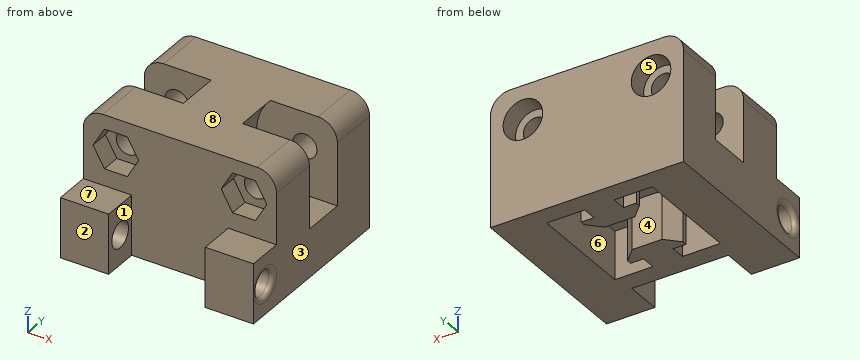
```python
from build123d import *

# Parameters (mm, degrees)
SKETCH1_W           = 40
SKETCH1_H           = 27
BOSS_EXTRUDE1_DEPTH = 30
CUT_EXTRUDE1_DEPTH  = 10
SKETCH3_R           = 2.5
CUT_EXTRUDE2_DEPTH  = 30
CUT_EXTRUDE5_START  = -10.62
CUT_EXTRUDE5_DEPTH  = 9
SKETCH10_W          = 20
SKETCH10_H          = 9
CUT_EXTRUDE7_DEPTH  = 6.8
SKETCH12_W          = 20
SKETCH12_H          = 9
CUT_EXTRUDE10_DEPTH = 6.8
FILLET1_R           = 4
SKETCH13_W          = 12.4
SKETCH13_H          = 7.4
SKETCH13_R          = 2.675
BOSS_EXTRUDE2_DEPTH = 40
CUT_EXTRUDE11_REACH = 42.436
SKETCH14_W          = 20
SKETCH14_H          = 7.4
SKETCH15_R          = 4.1
CUT_EXTRUDE12_DEPTH = 4
SKETCH16_R          = 2.5
CUT_EXTRUDE13_DEPTH = 4
FILLET2_SIZE        = 1


with BuildPart() as part:
    # Sketch1 → Boss-Extrude1 (new body)
    with BuildSketch(Plane(origin=(0, 0, 0), x_dir=(1, 0, 0), z_dir=(0, 1, 0))):
        with Locations((-2.846153846, 4.313186813)):
            Rectangle(SKETCH1_W, SKETCH1_H)
    extrude(amount=BOSS_EXTRUDE1_DEPTH)

    # Sketch2 → Cut-Extrude1 (cut)
    with BuildSketch(Plane(origin=(0, 0, -17.813186813), x_dir=(-1, 0, 0), z_dir=(0, 0, -1))):
        Polygon((-8.086431081, 26), (-8.086431081, 4), (-0.206431081, 4), (-0.206431081, 7), (-2.866431081, 7), (-2.866431081, 8.008707537), (-0.253846154, 10.628707537), (5.946153846, 10.628707537), (8.558738773, 8.008707537), (8.558738773, 7), (5.898738773, 7), (5.898738773, 4), (13.778738773, 4), (13.778738773, 26), (5.898738773, 26), (5.898738773, 23), (8.558738773, 23), (8.558738773, 21.991292463), (5.938738773, 19.378707537), (-0.246431081, 19.378707537), (-2.866431081, 21.991292463), (-2.866431081, 23), (-0.206431081, 23), (-0.206431081, 26), align=None)
    extrude(amount=-CUT_EXTRUDE1_DEPTH, mode=Mode.SUBTRACT)

    # Sketch3 → Cut-Extrude2 (cut)
    with BuildSketch(Plane.XZ):
        with Locations(Location((10.423846154, 2.186813187, 0), (0, 0, 270))):
            Circle(SKETCH3_R)
        with Locations(Location((-16.116153846, 2.186813187, 0), (0, 0, 90))):
            Circle(SKETCH3_R)
    extrude(amount=-CUT_EXTRUDE2_DEPTH, mode=Mode.SUBTRACT)

    # Sketch8 → Cut-Extrude5 (cut)
    with BuildSketch(Plane.XZ.offset(CUT_EXTRUDE5_START)):
        with BuildLine():
            Line((3.282417725, 9.186813187), (17.153846154, 9.186813187))
            Line((17.153846154, 9.186813187), (17.153846154, -7.813186813))
            Line((17.153846154, -7.813186813), (10.423846154, -7.813186813))
            ThreePointArc((10.423846154, -7.813186813), (1.204301697, -1.686170159), (3.282417725, 9.186813187))
        make_face()
        with BuildLine():
            Line((-22.846153846, -7.813186813), (-16.116153846, -7.813186813))
            ThreePointArc((-16.116153846, -7.813186813), (-6.896609389, -1.686170159), (-8.974725418, 9.186813187))
            Line((-8.974725418, 9.186813187), (-22.846153846, 9.186813187))
            Line((-22.846153846, 9.186813187), (-22.846153846, -7.813186813))
        make_face()
    extrude(amount=-CUT_EXTRUDE5_DEPTH, mode=Mode.SUBTRACT)

    # Sketch10 → Cut-Extrude7 (cut)
    with BuildSketch(Plane.ZY.offset(-8.086431081)):
        with Locations((-7.813186813, 15.12)):
            Rectangle(SKETCH10_W, SKETCH10_H)
    extrude(amount=CUT_EXTRUDE7_DEPTH, mode=Mode.SUBTRACT)

    # Sketch12 → Cut-Extrude10 (cut)
    with BuildSketch(Plane(origin=(-13.778738773, 0, 0), x_dir=(0, 0, -1), z_dir=(1, 0, 0))):
        with Locations((7.813186813, 15.12)):
            Rectangle(SKETCH12_W, SKETCH12_H)
    extrude(amount=CUT_EXTRUDE10_DEPTH, mode=Mode.SUBTRACT)

    # Fillet1
    fillet1_edges = [part.edges().sort_by_distance(p)[0] for p in [
        (17.153846154, 24.81, 9.186813187),
        (-22.846153846, 24.81, 9.186813187),
        (17.153846154, 5.31, 9.186813187),
        (-22.846153846, 5.31, 9.186813187),
    ]]
    fillet(fillet1_edges, radius=FILLET1_R)

    # Sketch13 → Boss-Extrude2 (add)
    with BuildSketch(Plane(origin=(17.153846154, 0, 0), x_dir=(0, 0, -1), z_dir=(1, 0, 0))):
        with Locations((11.613186813, -3.7)):
            Rectangle(SKETCH13_W, SKETCH13_H)
        with Locations((11.613186813, -3.7)):
            Circle(SKETCH13_R, mode=Mode.SUBTRACT)
    extrude(amount=-BOSS_EXTRUDE2_DEPTH)

    # Sketch14 → Cut-Extrude11 (cut, up to next)
    with BuildSketch(Plane.XY.offset(-5.413186813), mode=Mode.PRIVATE) as cut_extrude11_sk1:
        with Locations((-2.846153846, -3.7)):
            Rectangle(SKETCH14_W, SKETCH14_H)
    cut_extrude11_tool1 = extrude(cut_extrude11_sk1.sketch, amount=-CUT_EXTRUDE11_REACH, mode=Mode.PRIVATE) & part.part
    add(cut_extrude11_tool1.solids().sort_by_distance((-2.846154, -3.7, -5.413187))[0], mode=Mode.SUBTRACT)

    # Sketch15 → Cut-Extrude12 (cut)
    with BuildSketch(Plane(origin=(0, 30, 0), x_dir=(1, 0, 0), z_dir=(0, 1, 0))):
        with Locations(Location((-16.116153846, -2.186813187, 0), (0, 0, 270))):
            Circle(SKETCH15_R)
        with Locations(Location((10.423846154, -2.186813187, 0), (0, 0, 90))):
            Circle(SKETCH15_R)
    extrude(amount=-CUT_EXTRUDE12_DEPTH, mode=Mode.SUBTRACT)

    # Sketch16 → Cut-Extrude13 (cut)
    # profile 1 of 2: a face of its own
    with BuildSketch(Plane.XZ):
        Polygon((-13.749017742, -1.913186813), (-11.381881639, 2.186813187), (-13.749017742, 6.286813187), (-18.48328995, 6.286813187), (-20.850426054, 2.186813187), (-18.48328995, -1.913186813), align=None)
        with Locations(Location((-16.116153846, 2.186813187, 0), (0, 0, 270))):
            Circle(SKETCH16_R, mode=Mode.SUBTRACT)
    # profile 2 of 2: a face of its own
    with BuildSketch(Plane.XZ):
        Polygon((12.790982258, -1.913186813), (15.158118361, 2.186813187), (12.790982258, 6.286813187), (8.05671005, 6.286813187), (5.689573946, 2.186813187), (8.05671005, -1.913186813), align=None)
        with Locations(Location((10.423846154, 2.186813187, 0), (0, 0, 270))):
            Circle(SKETCH16_R, mode=Mode.SUBTRACT)
    extrude(amount=-CUT_EXTRUDE13_DEPTH, mode=Mode.SUBTRACT)

    # Fillet2
    # a fillet whose section is not a circle: 1 mm, written as the material it takes off along each edge
    with BuildSketch(Plane(origin=(-22.846153846, -3.7, -11.613186813), x_dir=(0, 0, -1), z_dir=(0, -1, 0))) as fillet2_piece_1:
        with BuildLine():
            Bezier((2.675, FILLET2_SIZE), (2.675, 0), (2.675 + FILLET2_SIZE, 0), weights=[1, 1, 1])
            Line((2.675 + FILLET2_SIZE, 0), (2.675, 0))
            Line((2.675, 0), (2.675, FILLET2_SIZE))
        make_face()
    revolve(axis=Axis((-22.846153846, -3.7, -11.613186813), (1, 0, 0)), mode=Mode.SUBTRACT)
    with BuildSketch(Plane(origin=(17.153846154, -3.7, -11.613186813), x_dir=(0, 0, -1), z_dir=(0, -1, 0))) as fillet2_piece_2:
        with BuildLine():
            Bezier((2.675, -FILLET2_SIZE), (2.675, 0), (2.675 + FILLET2_SIZE, 0), weights=[1, 1, 1])
            Line((2.675 + FILLET2_SIZE, 0), (2.675, 0))
            Line((2.675, 0), (2.675, -FILLET2_SIZE))
        make_face()
    revolve(axis=Axis((17.153846154, -3.7, -11.613186813), (1, 0, 0)), mode=Mode.SUBTRACT)


solid = part.part
```
Verification items for the finished model (mm, model axes). Face numbers are marked on the shaded views. A direction names the side the tool comes from. Coordinates: 2 decimals unless noted, no trailing zeros. Loops run counter-clockwise (first coordinate to the right, second up) from the corner with the lowest first, then second, coordinate; pieces in that order, holes last. Notation, with made-up numbers: (5, -35.75) -> (46, -35.75) arc R9 ccw to (46, -31.75) -> close; hole circle Ø11 at (-3.5, -14.75). An arc over 180 degrees is marked (long way). Answer in a Markdown table with one row per item.
1) Section check C-C (y = 5). Record the cut outline in (x, z), and give its area (3 significant figures).
The answers:
| item | result |
|---|---|
| outline | (-22.85, -17.81) -> (-13.78, -17.81) -> (-13.78, -7.81) -> (-5.9, -7.81) -> (-5.9, -17.81) -> (0.21, -17.81) -> (0.21, -7.81) -> (8.09, -7.81) -> (8.09, -17.81) -> (17.15, -17.81) -> (17.15, 5.19) arc R4 ccw to (13.15, 9.19) -> (-18.85, 9.19) arc R4 ccw to (-22.85, 5.19) -> close; hole circle Ø5 at (-16.12, 2.19); hole circle Ø5 at (10.42, 2.19) |
| area | 876 mm2 |
2) Draft check along X on the marked faces 1, 2, 3 and 4. Enter one of: released by +X, released by -X, zero draft, split by the parting line, or undercut.
The answers:
| item | result |
|---|---|
| face 1 | undercut |
| face 2 | zero draft |
| face 3 | released by +X |
| face 4 | undercut |
3) Section check A-A (y = 17). Record the cut outline in (x, z), and give its area (3 significant figures).
The answers:
| item | result |
|---|---|
| outline | (-22.85, -17.81) -> (-13.78, -17.81) -> (-13.78, -7.54) arc R10 cw to (-16.12, -7.81) -> (-22.85, -7.81) -> close; (-8.97, 9.19) arc R10 cw to (-6.98, -1.88) -> (-6.98, -7.81) -> (1.29, -7.81) -> (1.29, -1.88) arc R10 cw to (3.28, 9.19) -> close; (8.09, -17.81) -> (17.15, -17.81) -> (17.15, -7.81) -> (10.42, -7.81) arc R10 cw to (8.09, -7.54) -> close |
| area | 318 mm2 |
4) Section check D-D (z = -2.5). Record the cut outline in (x, y).
The answers:
| item | result |
|---|---|
| outline | (-22.85, 0) -> (17.15, 0) -> (17.15, 10.62) -> (1.29, 10.62) -> (1.29, 19.62) -> (17.15, 19.62) -> (17.15, 30) -> (-22.85, 30) -> (-22.85, 19.62) -> (-6.98, 19.62) -> (-6.98, 10.62) -> (-22.85, 10.62) -> close |
5) Depth check by flat-ended pin: P1, Ø4, axis at x = -0.5, z = -5.5, coming from the -Y side; P2, Ø8, axis at x = -16.12, z = 2.19, coming from the +Y side; P3, Ø3.5, axis at x = 12.5, y = 17, coming from the +Z side. Enter the tip coordinate at first touch or a pass-through.
The answers:
| item | result |
|---|---|
| P1 | stops at y = 0 |
| P2 | stops at y = 26 |
| P3 | stops at z = -7.81 |
6) Scan lines: line 1 along X through (y, z) = (5.5, -11); line 2 along Y through (x, z) = (-14.5, -7); line 3 along X through (y, z) = (28, 4). Record each from-to range of solid material in increasing order. Write a range as from..to.
The answers:
| item | result |
|---|---|
| line 1 | x = -22.85..-13.78, -5.9..0.21, 8.09..17.15 |
| line 2 | y = -7.4..10.62, 19.62..30 |
| line 3 | x = -22.85..-19.79, -12.44..6.75, 14.1..17.15 |
7) Section check B-B (x = -14.5). Record the cut outline in (y, z) (3 decimals).
The answers:
| item | result |
|---|---|
| outline | (-7.4, -17.813) -> (30, -17.813) -> (30, -1.581) -> (26, -1.581) -> (26, 0.279) -> (19.62, 0.279) -> (19.62, -7.682) -> (10.62, -7.682) -> (10.62, 0.279) -> (4, 0.279) -> (4, -1.913) -> (0, -1.913) -> (0, -5.413) -> (-7.4, -5.413) -> close; (0, 6.287) -> (4, 6.287) -> (4, 4.094) -> (10.62, 4.094) -> (10.62, 9.187) -> (0, 9.187) -> close; (19.62, 4.094) -> (26, 4.094) -> (26, 5.955) -> (30, 5.955) -> (30, 9.187) -> (19.62, 9.187) -> close; hole circle Ø5.35 at (-3.7, -11.613) |
8) Access from +Z, -Z, +X, -X, +Y, -Y to the whole of each face (thin tool, end or side, straight path). Record for the marked faces 5, 6, 7 and 8.
The answers:
| item | result |
|---|---|
| face 5 | +Y |
| face 6 | -Z |
| face 7 | +Z, +X, -X, -Y |
| face 8 | +Z, +X, -X, +Y, -Y |
